Answer from the drawing. Dimensions are ordinates in mm from the lowest x, y and z of the part. A direction names the side the tool comes from. Round coordinates to 2 decimals unless told otherwise and drop trailing zeros. Write each loop counter-clockwise with the first axis right and the second up, starting at its lowest first coordinate (ties: lowest second). Pieces come first, ordered by that corner, then holes. Notation, with made-up numbers: (81.5, 1) - (120.5, 1) arc R13 cw to (120.5, 13) - close; hole circle Ø8 at (-37.5, 55). An arc over 180 degrees is marked (long way). Use a Markdown table: item, result. Add a question column.
1) A cutting plane is placed at D-D (x = 116). Give the vertices of the cut face in (y, z).
2) A tool of negligible diameter and unlimited length cuts with its end or side. For the marked faces 5, 6 and 7, from which of +Z, -Z, +X, -X, +Y, -Y can it reach the whole face along a straight path? Write none if from no direction.
3) Find the intervals of material crossed by probe 1 along X at (y, z) = (63, 8); probe 2 along Y at (x, z) = (63.5, 3.75); probe 3 along Z at (x, y) = (105, 78.5), in increasing order. Write a range as from..to.
4) A cutting plane is placed at A-A (y = 63.5). Give the vertices of the cut face in (x, z).
5) Each of these flat-tipped pins is pushed along its axis until it touches: P1, Ø12, axis at x = 51, z = 56, coming from the -Y side; P2, Ø5, axis at y = 91.5, z = 37.5, coming from the +X side; P3, Ø3, axis at y = 44.5, z = 62.5, coming from the +X side. Where does it stop, or does it pass through?
6) Determine the mould class of the marked faces 1, 2, 3 and 4 for opening direction Z: +Z half, -Z half, draft (parallel to the pull), parting line (faces both ways), or undercut.
7) A cutting plane is placed at C-C (y = 9.5). Give the vertices of the cut face in (x, z), then the cut area to 3 significant figures.
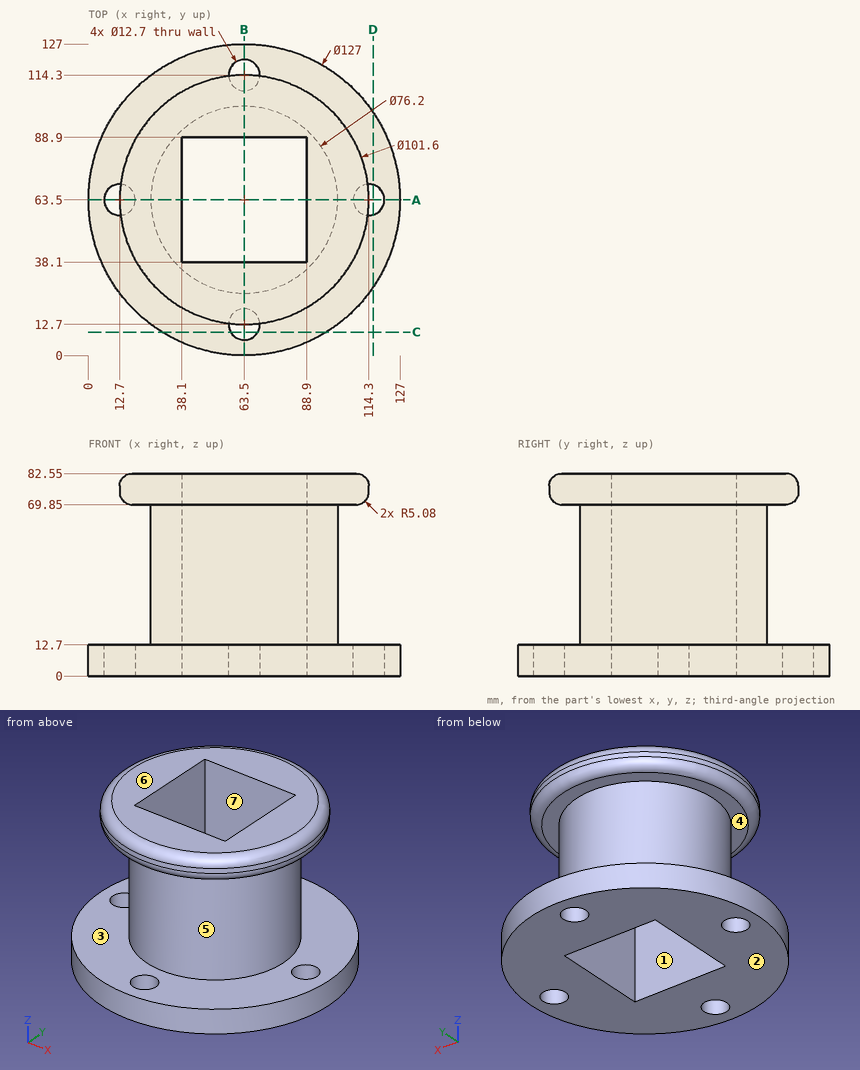
Entries:
| question | item | result |
|---|---|---|
| 1 | outline | (27.78, 0) - (57.38, 0) - (57.38, 12.7) - (27.78, 12.7) - close; (69.62, 0) - (99.22, 0) - (99.22, 12.7) - (69.62, 12.7) - close |
| 2 | face 5 | none |
| 2 | face 6 | +Z, +X, -X, +Y, -Y |
| 2 | face 7 | +Z, -Z |
| 3 | probe 1 | x = 0..6.37, 19.03..38.1, 88.9..107.97, 120.63..127 |
| 3 | probe 2 | y = 0..6.35, 19.05..38.1, 88.9..107.95, 120.65..127 |
| 3 | probe 3 | z = 0..12.7, 69.85..82.55 |
| 4 | outline | (0, 0) - (6.35, 0) - (6.35, 12.7) - (0, 12.7) - close; (12.7, 74.93) arc R5.08 ccw to (17.78, 69.85) - (25.4, 69.85) - (25.4, 12.7) - (19.05, 12.7) - (19.05, 0) - (38.1, 0) - (38.1, 82.55) - (17.78, 82.55) arc R5.08 ccw to (12.7, 77.47) - close; (88.9, 0) - (107.95, 0) - (107.95, 12.7) - (101.6, 12.7) - (101.6, 69.85) - (109.22, 69.85) arc R5.08 ccw to (114.3, 74.93) - (114.3, 77.47) arc R5.08 ccw to (109.22, 82.55) - (88.9, 82.55) - close; (120.65, 0) - (127, 0) - (127, 12.7) - (120.65, 12.7) - close |
| 5 | P1 | stops at y = 25.96 |
| 5 | P2 | stops at x = 91.81 |
| 5 | P3 | stops at x = 97.34 |
| 6 | face 1 | draft |
| 6 | face 2 | -Z half |
| 6 | face 3 | undercut |
| 6 | face 4 | undercut |
| 7 | outline | (30.09, 0) - (58.02, 0) - (58.02, 12.7) - (30.09, 12.7) - close; (68.98, 0) - (96.91, 0) - (96.91, 12.7) - (68.98, 12.7) - close |
| 7 | area | 709 mm² |
